Could you check a few things on this model? Use its own coordinates, in mm. A direction names the side the tool comes from. Give positions to 0.01 mm unless a question says otherwise; leave off trailing zeros. Order: outer loops, then holes, each group sorted by start corner. A loop starts at its lowest first (then second) coordinate and runs counter-clockwise, first axis right, second up. Notation, with made-up numbers: (16, -12) - (23, -12) arc R8 cw to (23, -4) - close; hole circle Ø6 at (40, 7). An arc over 180 degrees is marked (long way). One line per question, with ' | ' between items. Start each with the question number.
1. I need wall thicknesses on probe 1 along Z at (x, y) = (0.2, 3.25); probe 2 along Z at (x, y) = (1.4, 11.5); probe 3 along Y at (x, z) = (2.6, -35.5). Which ranges of each line are inside material? Lowest first, please. Write a range as from..to.
2. Imagine slicing it at A-A (y = 17). Please give me the cut outline in (x, z).
3. For P1, Ø1.5, axis at x = 1, y = 11, coming from the +Z side; P2, Ø1.4, axis at x = 2, y = 3.5, coming from the -Z side; P3, Ø1.5, axis at x = 1.5, z = -104.5, coming from the -Y side, each with a flat end and sliding along its axis, tell me the tip position at first contact or that it passes through.
4. Which directions (+Z, -Z, +X, -X, +Y, -Y) give clear straight access to the entire face, cutting with the end or side of a thin tool? Please do faces 1 (the flat face through (1, 3, -73.036)), 2 (the flat face through (1, 6.164, -43)), 3 (the flat face through (1, 4.564, -9)), 4 (the flat face through (1, 15.702, -8)), 5 (the flat face through (1, 10, -103.536)).
5. If we mould it in two halves opening along Y, with no side actions, what happens to faces 6 (the flat face through (1, 12.633, -1)), 7 (the flat face through (1, 7.633, -105)), 8 (the flat face through (1, 15.702, -53)), 9 (the flat face through (1, 3, -16.836))? For each: released by +Y, released by -Y, zero draft, split by the parting line, or undercut.
6. Imagine slicing it at C-C (y = 11.25). Please give me the cut outline in (x, z), and give its area (3 significant figures).
7. Imagine slicing it at B-B (z = -56). Please give me the cut outline in (x, y).
```python
from build123d import *

# Parameters (mm, degrees)
BOSS_EXTRUDE1_DEPTH = 3


with BuildPart() as part:
    # Sketch3 → Boss-Extrude1 (new body)
    with BuildSketch(Plane(origin=(0, 0, 0), x_dir=(0, 0, -1), z_dir=(1, 0, 0))):
        with BuildLine():
            Line((73.286325357, 18.701934502), (88.986325357, 18.701934502))
            ThreePointArc((88.986325357, 18.701934502), (89.163102052, 18.628711197), (89.236325357, 18.451934502))
            Line((89.236325357, 18.451934502), (89.236325357, 15.701934502))
            Line((89.236325357, 15.701934502), (105.886325357, 15.701934502))
            ThreePointArc((105.886325357, 15.701934502), (106.063102052, 15.628711197), (106.136325357, 15.451934502))
            Line((106.136325357, 15.451934502), (106.136325357, 12.883184502))
            ThreePointArc((106.136325357, 12.883184502), (106.063102052, 12.706407807), (105.886325357, 12.633184502))
            Line((105.886325357, 12.633184502), (104.036325357, 12.633184502))
            ThreePointArc((104.036325357, 12.633184502), (103.182771966, 12.986737893), (103.536325357, 12.133184502))
            Line((103.536325357, 12.133184502), (103.536325357, 8.133184502))
            ThreePointArc((103.536325357, 8.133184502), (103.182771966, 7.279631112), (104.036325357, 7.633184502))
            Line((104.036325357, 7.633184502), (105.886325357, 7.633184502))
            ThreePointArc((105.886325357, 7.633184502), (106.063102052, 7.559961197), (106.136325357, 7.383184502))
            Line((106.136325357, 7.383184502), (106.136325357, 4.814434502))
            ThreePointArc((106.136325357, 4.814434502), (106.063102052, 4.637657807), (105.886325357, 4.564434502))
            Line((105.886325357, 4.564434502), (89.236325357, 4.564434502))
            Line((89.236325357, 4.564434502), (89.236325357, 1.814434502))
            ThreePointArc((89.236325357, 1.814434502), (89.163102052, 1.637657807), (88.986325357, 1.564434502))
            Line((88.986325357, 1.564434502), (73.286325357, 1.564434502))
            ThreePointArc((73.286325357, 1.564434502), (73.109548661, 1.637657807), (73.036325357, 1.814434502))
            Line((73.036325357, 1.814434502), (73.036325357, 4.564434502))
            Line((73.036325357, 4.564434502), (33.036325357, 4.564434502))
            Line((33.036325357, 4.564434502), (33.036325357, 1.814434502))
            ThreePointArc((33.036325357, 1.814434502), (32.963102052, 1.637657807), (32.786325357, 1.564434502))
            Line((32.786325357, 1.564434502), (17.086325357, 1.564434502))
            ThreePointArc((17.086325357, 1.564434502), (16.909548661, 1.637657807), (16.836325357, 1.814434502))
            Line((16.836325357, 1.814434502), (16.836325357, 4.564434502))
            Line((16.836325357, 4.564434502), (0.186325357, 4.564434502))
            ThreePointArc((0.186325357, 4.564434502), (0.009548661, 4.637657807), (-0.063674643, 4.814434502))
            Line((-0.063674643, 4.814434502), (-0.063674643, 7.383184502))
            ThreePointArc((-0.063674643, 7.383184502), (0.009548661, 7.559961197), (0.186325357, 7.633184502))
            Line((0.186325357, 7.633184502), (2.436325357, 7.633184502))
            ThreePointArc((2.436325357, 7.633184502), (3.289878747, 7.279631112), (2.936325357, 8.133184502))
            Line((2.936325357, 8.133184502), (2.936325357, 12.133184502))
            ThreePointArc((2.936325357, 12.133184502), (3.289878747, 12.986737893), (2.436325357, 12.633184502))
            Line((2.436325357, 12.633184502), (0.186325357, 12.633184502))
            ThreePointArc((0.186325357, 12.633184502), (0.009548661, 12.706407807), (-0.063674643, 12.883184502))
            Line((-0.063674643, 12.883184502), (-0.063674643, 15.451934502))
            ThreePointArc((-0.063674643, 15.451934502), (0.009548661, 15.628711197), (0.186325357, 15.701934502))
            Line((0.186325357, 15.701934502), (16.836325357, 15.701934502))
            Line((16.836325357, 15.701934502), (16.836325357, 18.451934502))
            ThreePointArc((16.836325357, 18.451934502), (16.909548661, 18.628711197), (17.086325357, 18.701934502))
            Line((17.086325357, 18.701934502), (32.786325357, 18.701934502))
            ThreePointArc((32.786325357, 18.701934502), (32.963102052, 18.628711197), (33.036325357, 18.451934502))
            Line((33.036325357, 18.451934502), (33.036325357, 15.701934502))
            Line((33.036325357, 15.701934502), (73.036325357, 15.701934502))
            Line((73.036325357, 15.701934502), (73.036325357, 18.451934502))
            ThreePointArc((73.036325357, 18.451934502), (73.109548661, 18.628711197), (73.286325357, 18.701934502))
        make_face()
        with BuildLine():
            Line((37.136325357, 6.164434502), (48.636325357, 6.164434502))
            ThreePointArc((48.636325357, 6.164434502), (48.813102052, 6.237657807), (48.886325357, 6.414434502))
            Line((48.886325357, 6.414434502), (48.886325357, 8.414434502))
            ThreePointArc((48.886325357, 8.414434502), (48.813102052, 8.591211197), (48.636325357, 8.664434502))
            Line((48.636325357, 8.664434502), (37.136325357, 8.664434502))
            ThreePointArc((37.136325357, 8.664434502), (36.959548661, 8.591211197), (36.886325357, 8.414434502))
            Line((36.886325357, 8.414434502), (36.886325357, 6.414434502))
            ThreePointArc((36.886325357, 6.414434502), (36.959548661, 6.237657807), (37.136325357, 6.164434502))
        make_face(mode=Mode.SUBTRACT)
    extrude(amount=BOSS_EXTRUDE1_DEPTH)


solid = part.part
```
Results found:
1) probe 1: z = -89.24..-73.04, -33.04..-16.84 | probe 2: z = -103.54..-2.94 | probe 3: y = 4.56..15.7
2) outline: (0, -89.24) - (3, -89.24) - (3, -73.04) - (0, -73.04) - close; (0, -33.04) - (3, -33.04) - (3, -16.84) - (0, -16.84) - close
3) P1: stops at z = -2.94 | P2: stops at z = -89.24 | P3: stops at y = 4.56
4) face 1: +X, -X, -Y | face 2: +X, -X | face 3: +Z, +X, -X, -Y | face 4: +Z, +X, -X, +Y | face 5: -Z, +X, -X
5) face 6: undercut | face 7: undercut | face 8: released by +Y | face 9: zero draft
6) outline: (0, -103.54) - (3, -103.54) - (3, -2.94) - (0, -2.94) - close | area: 302 mm2
7) outline: (0, 4.56) - (3, 4.56) - (3, 15.7) - (0, 15.7) - close
